from build123d import *

# Parameters (mm, degrees)
F0_W     = 406.4
F0_H     = 812.8
F0_W_2   = 330.2
F0_H_2   = 38.1
F1_DEPTH = 38.1


with BuildPart() as f1:
    # F0 (on Front) → F1 (new body)
    with BuildSketch(Plane.XZ):
        Rectangle(F0_W, F0_H)
        Polygon((165.1, -19.05), (165.1, -368.3), (-165.1, -368.3), (-165.1, -19.05), (-165.1, 19.05), (-165.1, 368.3), (165.1, 368.3), (165.1, 19.05), align=None, mode=Mode.SUBTRACT)
        Rectangle(F0_W_2, F0_H_2)
    extrude(amount=F1_DEPTH)


solid = f1.part
Design review of the part built by this model. Coordinates are the model's own, in mm. A direction names the side the tool comes from. Coordinates: 2 decimals unless noted, no trailing zeros. Write each loop counter-clockwise with the first axis right and the second up, starting at its lowest first coordinate (ties: lowest second). Pieces come first, ordered by that corner, then holes. Notation, with made-up numbers: (42.25, -13) - (83.25, -13) arc R12 ccw to (83.25, -4) - close; hole circle Ø11 at (38, 51). An arc over 180 degrees is marked (long way). Use one line per item in the form item = value.
Q1. Consider section C-C (y = -23). Write out the cut boundary in (x, z), plus the area to 3 significant figures.
Taken from the geometry:
outline = (-203.2, -406.4) - (203.2, -406.4) - (203.2, 406.4) - (-203.2, 406.4) - close; hole (-165.1, -368.3) - (165.1, -368.3) - (165.1, -19.05) - (-165.1, -19.05) - close; hole (-165.1, 19.05) - (165.1, 19.05) - (165.1, 368.3) - (-165.1, 368.3) - close
area = 99,700 mm^2
Q2. Consider section B-B (z = -80). Write out the cut boundary in (x, y), plus the area to 3 significant figures.
Taken from the geometry:
outline = (-203.2, -38.1) - (-165.1, -38.1) - (-165.1, 0) - (-203.2, 0) - close; (165.1, -38.1) - (203.2, -38.1) - (203.2, 0) - (165.1, 0) - close
area = 2,900 mm^2
Q3. The part is to be moulded in two halves that separate along Z. For faces 1 (the flat face through (165.1, -19, -191)), 2 (the flat face through (-1, -38.1, 2)), 3 (the flat face through (-3, -19, -406.4)), 4 (the flat face through (-2, -19, 368.3)), say which applies: +Z half, -Z half, draft (parallel to the pull), parting line (faces both ways), or undercut.
Taken from the geometry:
face_1 = undercut
face_2 = draft
face_3 = -Z half
face_4 = undercut
Q4. For probe 1 along Z at (x, y) = (-39, -19.5); probe 2 along X at (y, z) = (-14, 332), list the stretches that pass through material, from the lowest coordinate up.
Taken from the geometry:
probe_1 = -406.4 to -368.3, -19.05 to 19.05, 368.3 to 406.4
probe_2 = -203.2 to -165.1, 165.1 to 203.2
Q5. Machinability: for faces 5 (the flat face through (-3, -19, 406.4)), 6 (the flat face through (2, -19, -368.3)), which of the approach directions +Z, -Z, +X, -X, +Y, -Y give a long, thin tool a straight path to every point of the face, cutting with its end or side? Answer none if there is none.
Taken from the geometry:
face_5 = +Z, +X, -X, +Y, -Y
face_6 = +Y, -Y
Q6. Consider section A-A (x = -96.5). Write out the cut boundary in (y, z), plus the area to 3 significant figures.
Taken from the geometry:
outline = (-38.1, -406.4) - (0, -406.4) - (0, -368.3) - (-38.1, -368.3) - close; (-38.1, -19.05) - (0, -19.05) - (0, 19.05) - (-38.1, 19.05) - close; (-38.1, 368.3) - (0, 368.3) - (0, 406.4) - (-38.1, 406.4) - close
area = 4,350 mm^2
